from build123d import *

# Parameters (mm, degrees)
SKETCH1_W           = 130
SKETCH1_H           = 6
SKETCH1_W_2         = 5.5
SKETCH1_H_2         = 5.5
BOSS_EXTRUDE1_DEPTH = 232


with BuildPart() as part:
    # Sketch1 → Boss-Extrude1 (new body)
    with BuildSketch(Plane(origin=(0, 0, 0), x_dir=(1, 0, 0), z_dir=(0, 1, 0))):
        with Locations((65, 3)):
            Rectangle(SKETCH1_W, SKETCH1_H)
        with Locations((8.75, 3)):
            Rectangle(SKETCH1_W_2, SKETCH1_H_2, mode=Mode.SUBTRACT)
        with Locations((3, 3)):
            Rectangle(SKETCH1_W_2, SKETCH1_H_2, mode=Mode.SUBTRACT)
        with Locations((14.5, 3)):
            Rectangle(SKETCH1_W_2, SKETCH1_H_2, mode=Mode.SUBTRACT)
        with Locations((20.25, 3)):
            Rectangle(SKETCH1_W_2, SKETCH1_H_2, mode=Mode.SUBTRACT)
        with Locations((26, 3)):
            Rectangle(SKETCH1_W_2, SKETCH1_H_2, mode=Mode.SUBTRACT)
        with Locations((31.75, 3)):
            Rectangle(SKETCH1_W_2, SKETCH1_H_2, mode=Mode.SUBTRACT)
        with Locations((37.5, 3)):
            Rectangle(SKETCH1_W_2, SKETCH1_H_2, mode=Mode.SUBTRACT)
        with Locations((43.25, 3)):
            Rectangle(SKETCH1_W_2, SKETCH1_H_2, mode=Mode.SUBTRACT)
        with Locations((49, 3)):
            Rectangle(SKETCH1_W_2, SKETCH1_H_2, mode=Mode.SUBTRACT)
        with Locations((54.75, 3)):
            Rectangle(SKETCH1_W_2, SKETCH1_H_2, mode=Mode.SUBTRACT)
        with Locations((60.5, 3)):
            Rectangle(SKETCH1_W_2, SKETCH1_H_2, mode=Mode.SUBTRACT)
        with Locations((66.25, 3)):
            Rectangle(SKETCH1_W_2, SKETCH1_H_2, mode=Mode.SUBTRACT)
        with Locations((72, 3)):
            Rectangle(SKETCH1_W_2, SKETCH1_H_2, mode=Mode.SUBTRACT)
        with Locations((77.75, 3)):
            Rectangle(SKETCH1_W_2, SKETCH1_H_2, mode=Mode.SUBTRACT)
        with Locations((83.5, 3)):
            Rectangle(SKETCH1_W_2, SKETCH1_H_2, mode=Mode.SUBTRACT)
        with Locations((89.25, 3)):
            Rectangle(SKETCH1_W_2, SKETCH1_H_2, mode=Mode.SUBTRACT)
        with Locations((95, 3)):
            Rectangle(SKETCH1_W_2, SKETCH1_H_2, mode=Mode.SUBTRACT)
        with Locations((100.75, 3)):
            Rectangle(SKETCH1_W_2, SKETCH1_H_2, mode=Mode.SUBTRACT)
        with Locations((106.5, 3)):
            Rectangle(SKETCH1_W_2, SKETCH1_H_2, mode=Mode.SUBTRACT)
        with Locations((112.25, 3)):
            Rectangle(SKETCH1_W_2, SKETCH1_H_2, mode=Mode.SUBTRACT)
        with Locations((118, 3)):
            Rectangle(SKETCH1_W_2, SKETCH1_H_2, mode=Mode.SUBTRACT)
        with Locations((123.75, 3)):
            Rectangle(SKETCH1_W_2, SKETCH1_H_2, mode=Mode.SUBTRACT)
    extrude(amount=BOSS_EXTRUDE1_DEPTH)


solid = part.part
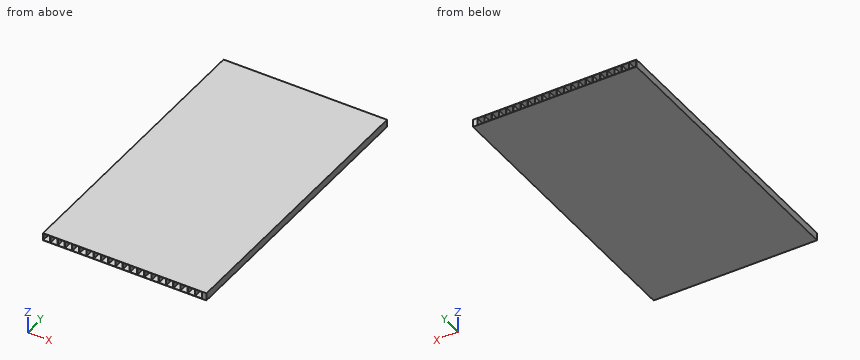
The model under review builds one solid part; all positions refer to its coordinate system, in mm. Round coordinates to 2 decimals unless told otherwise and drop trailing zeros. Write each loop counter-clockwise with the first axis right and the second up, starting at its lowest first coordinate (ties: lowest second). Pieces come first, ordered by that corner, then holes. Notation, with made-up numbers: M 88,-39 L 132,-39 A19 ccw 132,-31 Z; hole C -13,-3 d10. An arc over 180 degrees is marked long. Use a Markdown table: item, result. Add a question column.
Q1. We need section A-A, the plane x = 14. State the section outline as (y, z) points, plus the area to 3 significant figures.
Q2. We need section B-B, the plane z = -4.2. Count the separate pieces of the cut face and the enclosed holes in it, plus the area to 3 significant figures.
Q3. To check wall thickness, follow line 1 (Z direction, x = 51.5, y = 149.5). State the ranges of the line that lie inside material, in increasing order.
Findings below:
| question | item | result |
|---|---|---|
| 1 | outline | M 0,-6 L 232,-6 L 232,-5.75 L 0,-5.75 Z; M 0,-0.25 L 232,-0.25 L 232,0 L 0,0 Z |
| 1 | area | 116 mm² |
| 2 | separate pieces | 23 |
| 2 | enclosed holes | 0 |
| 2 | area | 2,090 mm² |
| 3 | line 1 | z = -6 to -5.75, -0.25 to 0 |
